from build123d import *

# Parameters (mm, degrees)
SKETCH1_R           = 30
BOSS_EXTRUDE1_DEPTH = 7.5
BOSS_EXTRUDE2_DEPTH = 15
SKETCH4_R           = 20
BOSS_EXTRUDE3_DEPTH = 18
CUT_EXTRUDE1_DEPTH  = 37
CIRPATTERN1_COUNT   = 16


with BuildPart() as part:
    # Sketch1 → Boss-Extrude1 (new body, symmetric)
    with BuildSketch(Plane(origin=(0, 0, 0), x_dir=(0, 0, -1), z_dir=(1, 0, 0))):
        Circle(SKETCH1_R)
    extrude(amount=BOSS_EXTRUDE1_DEPTH, both=True)

    # Sketch3 → Boss-Extrude2 (add)
    with BuildSketch(Plane(origin=(7.5, 0, 0), x_dir=(0, 0, -1), z_dir=(1, 0, 0))):
        with BuildLine():
            Line((-1.5, 35.732137495), (1.5, 35.732137495))
            ThreePointArc((1.5, 35.732137495), (3.203300204, 32.92101258), (4, 29.732137495))
            ThreePointArc((4, 29.732137495), (0, 30), (-4, 29.732137495))
            ThreePointArc((-4, 29.732137495), (-3.203300204, 32.92101258), (-1.5, 35.732137495))
        make_face()
    boss_extrude2 = extrude(amount=-BOSS_EXTRUDE2_DEPTH)

    # Sketch4 → Boss-Extrude3 (add, symmetric)
    with BuildSketch(Plane(origin=(0, 0, 0), x_dir=(0, 0, -1), z_dir=(1, 0, 0))):
        Circle(SKETCH4_R)
    extrude(amount=BOSS_EXTRUDE3_DEPTH, both=True)

    # Sketch5 → Cut-Extrude1 (cut, through all)
    with BuildSketch(Plane(origin=(18, 0, 0), x_dir=(0, 0, -1), z_dir=(1, 0, 0))):
        with BuildLine():
            Line((-4, 15), (4, 15))
            Line((4, 15), (4, 11.842719282))
            ThreePointArc((4, 11.842719282), (0, -12.5), (-4, 11.842719282))
            Line((-4, 11.842719282), (-4, 15))
        make_face()
    extrude(amount=-CUT_EXTRUDE1_DEPTH, mode=Mode.SUBTRACT)

    # CirPattern1: Boss-Extrude2 ×16 about axis
    cirpattern1_axis = Axis((0, 0, 0), (1, 0, 0))
    for i in range(1, CIRPATTERN1_COUNT):
        add(boss_extrude2.rotate(cirpattern1_axis, i * 360 / CIRPATTERN1_COUNT))


solid = part.part
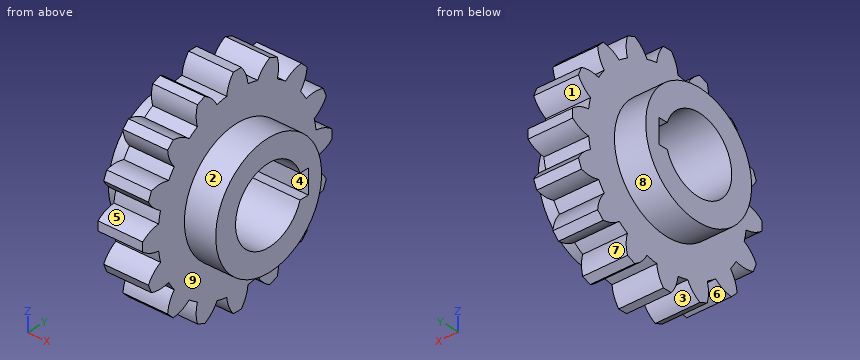
Verification items for the finished model (mm, model axes). Face numbers are marked on the shaded views. A direction names the side the tool comes from. Give positions to 0.01 mm unless a question says otherwise; leave off trailing zeros. Write each loop counter-clockwise with the first axis right and the second up, starting at its lowest first coordinate (ties: lowest second). Pieces come first, ordered by that corner, then holes. Notation, with made-up numbers: M -32.5,68.5 L -19.5,68.5 A23 cw -19.5,87.5 Z; hole C 4.5,3.25 d10. An arc over 180 degrees is marked long. Write item = value, one per line.
(1) Go/stop test with flat-tipped pins: pin 1 Ø6 at (x, z) = (-8, 22.5) entering from -Y; pin 2 Ø8 at (x, y) = (6.5, 20.5) entering from -Z; pin 3 Ø3.5 at (x, y) = (0.5, 12.5) entering from +Z. Record where each tip stops, or that it passes through.
Found:
pin_1 = -26.33
pin_2 = -26.33
pin_3 = 33.59
(2) Sectioned sample at A-A (y = 0). Record the cut outline in (x, z), then the cut area to 3 significant figures.
Found:
outline = M -18,-20 L -7.5,-20 L -7.5,-35.73 L 7.5,-35.73 L 7.5,-20 L 18,-20 L 18,-12.5 L -18,-12.5 Z; M -18,12.5 L 18,12.5 L 18,20 L 7.5,20 L 7.5,35.73 L -7.5,35.73 L -7.5,20 L -18,20 Z
area = 1,010 mm2
(3) Access from +Z, -Z, +X, -X, +Y, -Y to the whole of each face (thin tool, end or side, straight path). Record for the marked faces 1, 2, 3, 4 and 5.
Found:
face_1 = +X, -X, +Y
face_2 = +X
face_3 = -Z, +X, -X
face_4 = +X, -X
face_5 = +X, -X, -Y
(4) Sectioned sample at B-B (z = 0). Record the cut outline in (x, y), then the cut area to 3 significant figures.
Found:
outline = M -18,-20 L -7.5,-20 L -7.5,-35.73 L 7.5,-35.73 L 7.5,-20 L 18,-20 L 18,-12.5 L -18,-12.5 Z; M -18,15 L 18,15 L 18,20 L 7.5,20 L 7.5,35.73 L -7.5,35.73 L -7.5,20 L -18,20 Z
area = 922 mm2
(5) Draft check along Z on the marked faces 6, 7, 8 and 9. Enter one of: released by +Z, released by -Z, zero draft, split by the parting line, or undercut.
Found:
face_6 = released by -Z
face_7 = undercut
face_8 = split by the parting line
face_9 = zero draft
(6) Sectioned sample at C-C (x = 13). Record the cut outline in (y, z).
Found:
outline = C 0,0 d40; hole M 11.84,-4 L 15,-4 L 15,4 L 11.84,4 A12.5 ccw long Z
(7) Material ranges on line 1 (Z direction, x = 5, y = 0); line 2 (Y direction, x = 8, z = 0); line 3 (Y direction, x = 6, z = 0), recorded low to high.
Found:
line_1 = -35.73 to -12.5, 12.5 to 35.73
line_2 = -20 to -12.5, 15 to 20
line_3 = -35.73 to -12.5, 15 to 35.73
